The listing builds one solid part. Answer for the finished solid, in the listing's coordinates (mm). Face numbers are marked on the shaded views. A direction names the side the tool comes from. Give positions to 0.01 mm unless a question says otherwise; leave off trailing zeros. Write each loop counter-clockwise with the first axis right and the second up, starting at its lowest first coordinate (ties: lowest second). Pieces come first, ordered by that corner, then holes. Notation, with made-up numbers: (-29, -18) - (15, -18) arc R22 ccw to (15, 16) - close; hole circle Ø8 at (-16.75, -14). An arc over 180 degrees is marked (long way). One line per item, written item: value. Start each with the question number.
from build123d import *

# Parameters (mm, degrees)
F0_R     = 68
F0_R_2   = 8.5
F1_DEPTH = 100
F2_DEPTH = 9
F4_R     = 2.5
F5_DEPTH = 75
F6_R     = 2.5
F7_DEPTH = 75
F3_R     = 7
F8_DEPTH = 18


with BuildPart() as f1:
    # F0 (on Front) → F1 (new body)
    with BuildSketch(Plane.XZ):
        Circle(F0_R)
        Circle(F0_R_2, mode=Mode.SUBTRACT)
        Circle(F0_R_2)
    extrude(amount=F1_DEPTH)

    # F0 (on Front) → F2 (join)
    with BuildSketch(Plane.XZ):
        Circle(F0_R_2)
    extrude(amount=-F2_DEPTH)

    # F4 (on Top) → F5 (cut, symmetric)
    with BuildSketch(Plane.XY):
        with Locations((0, -20.5)):
            Circle(F4_R)
    extrude(amount=F5_DEPTH, both=True, mode=Mode.SUBTRACT)

    # F6 (on Right) → F7 (cut, symmetric)
    with BuildSketch(Plane.YZ):
        with Locations((-20.5, 0)):
            Circle(F6_R)
    extrude(amount=F7_DEPTH, both=True, mode=Mode.SUBTRACT)

    # F3 (on face) → F8 (join)
    with BuildSketch(Plane(origin=(0, 9, 0), x_dir=(-1, 0, 0), z_dir=(0, 1, 0))):
        Circle(F3_R)
    extrude(amount=F8_DEPTH)


solid = f1.part
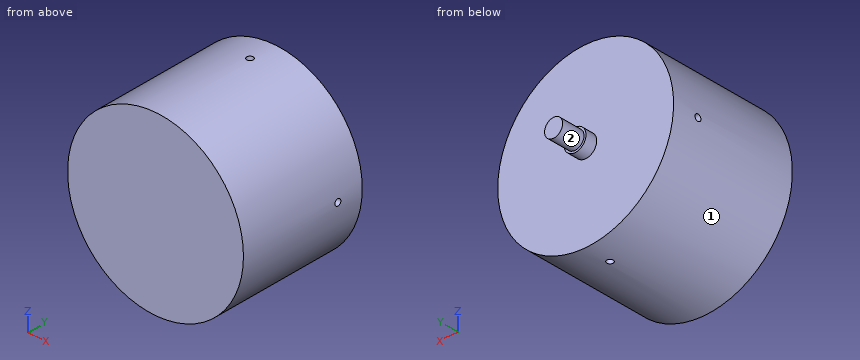
Item 1: Find section A-A on z = -17.5. Determine the outline of the cut face in (x, y), plus the area to 3 significant figures.
Item 2: For the marked faces 1 and 2, determine the directions among +Z, -Z, +X, -X, +Y, -Y from which every point of the face is accessible in a straight line to the end or side of a thin tool.
Item 3: Each of these flat-tipped pins is pushed along its axis until it touches: pin 1 Ø6 at (x, z) = (-4.5, 26.5) entering from +Y; pin 2 Ø6 at (y, z) = (-52, -50.5) entering from +X; pin 3 Ø1.5 at (y, z) = (-1.5, -41.5) entering from -X; pin 4 Ø6 at (x, y) = (0, -20.5) entering from +Z. Where does it stop, or does it pass through?
Item 4: Find section C-C on x = 24. Determine the outline of the cut face in (y, z).
Item 5: Find section D-D on y = -75.5. Determine the outline of the cut face in (x, z), plus the area to 3 significant figures.
Item 6: Straight lines are drawn through the part: line 1 along Y through (x, z) = (22, 0); line 2 along Y through (x, z) = (-42.5, -24); line 3 along Y through (x, z) = (3, 0). For each, find the intervals that lie inside material, in ascending order.
Item 7: Find section B-B on y = -20.5. Determine the outline of the cut face in (x, z), plus the area to 3 significant figures.
Values:
1. outline: (-65.71, -100) - (65.71, -100) - (65.71, 0) - (-65.71, 0) - close; hole circle Ø5 at (0, -20.5)
1. area: 13,100 mm^2
2. face 1: +Y, -Y
2. face 2: +Y
3. pin 1: y = 0
3. pin 2: x = 48.66
3. pin 3: x = -54.44
3. pin 4: z = 68
4. outline: (-100, -63.62) - (0, -63.62) - (0, 63.62) - (-100, 63.62) - close; hole circle Ø5 at (-20.5, 0)
5. outline: circle Ø136 at (0, 0)
5. area: 14,500 mm^2
6. line 1: -100 to -23, -18 to 0
6. line 2: -100 to 0
6. line 3: -100 to -23, -18 to 27
7. outline: (-67.95, -2.5) arc R68 ccw to (-2.5, -67.95) - (-2.5, -2.5) - close; (-67.95, 2.5) - (-2.5, 2.5) - (-2.5, 67.95) arc R68 ccw to start; (2.5, -67.95) arc R68 ccw to (67.95, -2.5) - (2.5, -2.5) - close; (2.5, 2.5) - (67.95, 2.5) arc R68 ccw to (2.5, 67.95) - close
7. area: 13,200 mm^2
